Could you check a few things on this drawing? It's one solid part, dimensions in mm from its lowest x, y, z. A direction names the side the tool comes from. Give positions to 0.01 mm unless a question says otherwise; leave off trailing zeros. Order: outer loops, then holes, each group sorted by start corner. A loop starts at its lowest first (then second) coordinate and runs counter-clockwise, first axis right, second up.
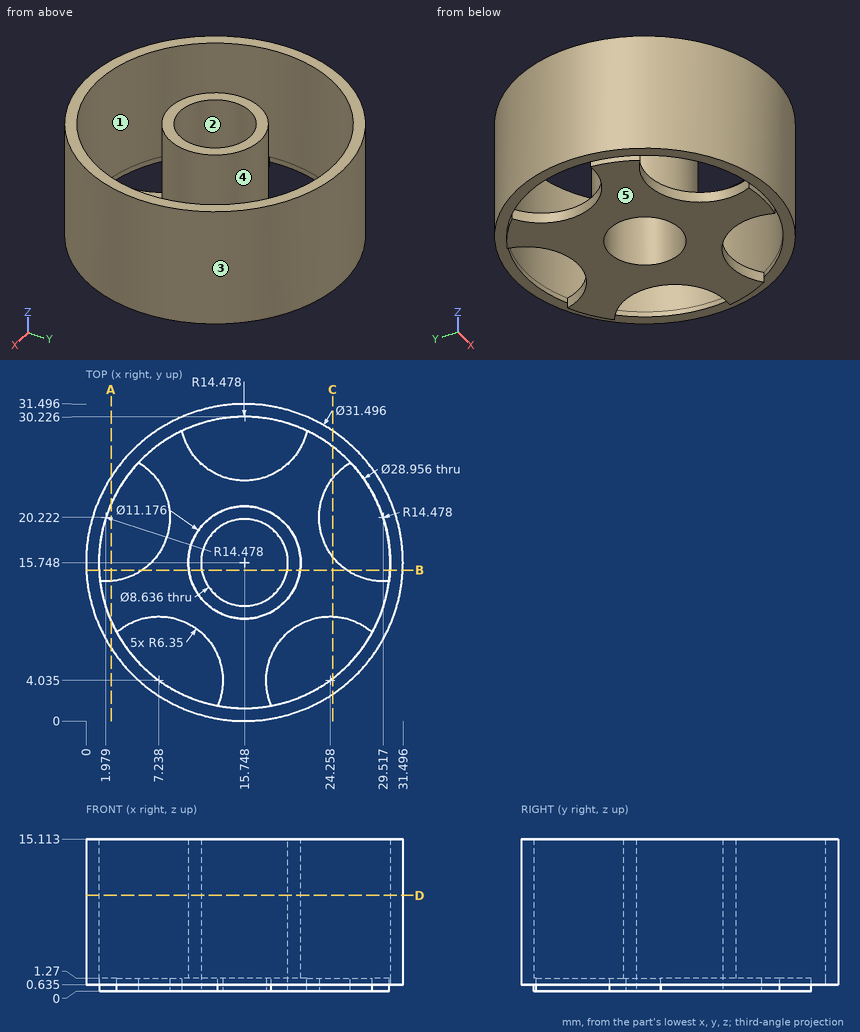
Q1. For the marked faces 1 and 2, which set-ups out of +Z, -Z, +X, -X, +Y, -Y let a thin tool reach every point of the face, with its end or its side?
Filled sheet:
face 1: +Z
face 2: +Z, -Z
Q2. I'm going to push flat-ended pins straight in: P1, Ø2, axis at y = 17.5, z = 5, coming from the -X side; P2, Ø1.5, axis at y = 9, z = 5.5, coming from the -X side; P3, Ø4, axis at x = 7, z = 3, coming from the -Y side. Where does each tip first touch, or does it pass through?
Filled sheet:
P1: stops at x = 0.02
P2: stops at x = 1.19
P3: stops at y = 1.52
Q3. If we section it at A-A on x = 2.5: List the corners of the cut face in (y, z) for me (1 decimal).
Filled sheet:
outline: (7.2, 0.6) - (9.9, 0.6) - (9.9, 0) - (13.9, 0) - (13.9, 1.3) - (9.9, 1.3) - (9.9, 15.1) - (7.2, 15.1) - close; (21.6, 0.6) - (24.3, 0.6) - (24.3, 15.1) - (21.6, 15.1) - close
Q4. Thinking about a two-plate mould opening in X: for the marked faces 3, 4 and 5, which applies, released by +X, released by -X, zero draft, split by the parting line, or undercut?
Filled sheet:
face 3: split by the parting line
face 4: undercut
face 5: zero draft
Q5. If we section it at C-C on x = 24.5: List the corners of the cut face in (y, z) for me (1 decimal).
Filled sheet:
outline: (2.7, 0.6) - (4.2, 0.6) - (4.2, 15.1) - (2.7, 15.1) - close; (10.4, 0) - (16.3, 0) - (16.3, 1.3) - (10.4, 1.3) - close; (24.1, 0) - (27.3, 0) - (27.3, 0.6) - (28.8, 0.6) - (28.8, 15.1) - (27.3, 15.1) - (27.3, 1.3) - (24.1, 1.3) - close
Q6. If we section it at B-B on y = 15: List the corners of the cut face in (x, z) for me (1 decimal).
Filled sheet:
outline: (0, 0.6) - (1.3, 0.6) - (1.3, 15.1) - (0, 15.1) - close; (5.6, 0) - (11.5, 0) - (11.5, 15.1) - (10.2, 15.1) - (10.2, 1.3) - (5.6, 1.3) - close; (20, 0) - (25.9, 0) - (25.9, 1.3) - (21.3, 1.3) - (21.3, 15.1) - (20, 15.1) - close; (30.2, 0.6) - (31.5, 0.6) - (31.5, 15.1) - (30.2, 15.1) - close
Q7. If we section it at D-D on z = 9.5: List the corners of the cut face in (x, y) for me, plus the area to 3 significant figures.
Filled sheet:
outline: circle Ø31.5 at (15.75, 15.75); circle Ø11.18 at (15.75, 15.75); hole circle Ø28.96 at (15.75, 15.75); hole circle Ø8.64 at (15.75, 15.75)
area: 160 mm2
Q8. I need wall thicknesses on L1, parallel to X at y = 18.5, z = 1 (1 decimal); L2, parallel to X at y = 23, z = 1 (1 decimal); L3, parallel to X at y = 19, z = 14.5 (1 decimal). Which ranges of each line are inside material? Lowest first, please.
Filled sheet:
L1: x = 0.2 to 1.5, 8.1 to 12.4, 19.1 to 23.4, 30 to 31.3
L2: x = 1.8 to 3.2, 7.7 to 23.8, 28.3 to 29.7
L3: x = 0.3 to 1.6, 11.2 to 12.9, 18.6 to 20.3, 29.9 to 31.2
